Could you check a few things on this model? Use its own coordinates, in mm. A direction names the side the tool comes from. Give positions to 0.01 mm unless a question says otherwise; leave off trailing zeros. Write each loop counter-clockwise with the first axis right and the second up, starting at its lowest first coordinate (ties: lowest second). Pieces come first, ordered by that corner, then holes. Notation, with made-up numbers: M 68.25,-28 L 110.25,-28 A16 ccw 110.25,-9 Z; hole C 88.25,20 d8. An arc over 180 degrees is marked long. One line per item, written item: value.
```python
from build123d import *

# Parameters (mm, degrees)
BOSS_EXTRUDE1_DEPTH      = 180
SKETCH3_W                = 116.5
SKETCH3_H                = 142
CUT_REVOLVE1_ANGLE       = 271
WRAP1_SECTION_W          = 10
WRAP1_SECTION_H          = 10
WRAP1_ANGLE              = 2.220766648
WRAP1_SECTOR_2_SECTION_W = 10
WRAP1_SECTOR_2_SECTION_H = 10
WRAP1_SECTOR_2_ANGLE     = 2.220766648
MIRROR1_START            = 60
MIRROR1_DEPTH            = 10
MIRROR1_START_2          = 110
MIRROR1_2_DEPTH          = 10
CUT_EXTRUDE6_DEPTH       = 262.461278204
CUT_EXTRUDE6_DEPTH_BACK  = 20
SKETCH17_R               = 2
CUT_EXTRUDE7_DEPTH       = 10
CUT_EXTRUDE9_DEPTH       = 262.461278204
CUT_EXTRUDE9_DEPTH_BACK  = 262.461278204
SKETCH19_W               = 258
SKETCH19_H               = 15.225908702
CUT_EXTRUDE10_DEPTH      = 252.222015682
CUT_EXTRUDE10_DEPTH_BACK = 252.222015682
SKETCH22_W               = 258
SKETCH22_H               = 14
SKETCH22_H_2             = 3.774091298


# Read off the part's stored shape, not the designer's step: Mirror1
with BuildPart() as part:
    # Sketch1 → Boss-Extrude1 (new body)
    with BuildSketch(Plane(origin=(0, 0, 0), x_dir=(1, 0, 0), z_dir=(0, 1, 0))):
        with BuildLine():
            Line((0, -129), (0, 129))
            ThreePointArc((0, 129), (-129, 0), (0, -129))
        make_face()
    extrude(amount=BOSS_EXTRUDE1_DEPTH)

    # Sketch3 → Cut-Revolve1 (revolve, cut)
    with BuildSketch(Plane(origin=(0, 0, 0), x_dir=(0, 0, -1), z_dir=(1, 0, 0))):
        with Locations((-58.25, 90)):
            Rectangle(SKETCH3_W, SKETCH3_H)
    revolve(axis=Axis((0, 180, 0), (0, -1, 0)), revolution_arc=CUT_REVOLVE1_ANGLE, mode=Mode.SUBTRACT)

    # Wrap1 section (on wrap section) → Wrap1 (revolve)
    with BuildSketch(Plane(origin=(0, 0, 0), x_dir=(0, 0, 1), z_dir=(1, 0, 0))):
        with Locations((134, -115)):
            Rectangle(WRAP1_SECTION_W, WRAP1_SECTION_H)
    revolve(axis=Axis((0, 0, 0), (0, -1, 0)), revolution_arc=WRAP1_ANGLE)

    # Wrap1 sector 2 section (on wrap section) → Wrap1 sector 2 (revolve)
    with BuildSketch(Plane(origin=(0, 0, 0), x_dir=(0, 0, 1), z_dir=(1, 0, 0))):
        with Locations((134, -65)):
            Rectangle(WRAP1_SECTOR_2_SECTION_W, WRAP1_SECTOR_2_SECTION_H)
    revolve(axis=Axis((0, 0, 0), (0, -1, 0)), revolution_arc=WRAP1_SECTOR_2_ANGLE)

    # Mirror1 outline → Mirror1 (add)
    with BuildSketch(Plane(origin=(0, 0, 0), x_dir=(1, 0, 0), z_dir=(0, 1, 0)).offset(MIRROR1_START)):
        with BuildLine():
            ThreePointArc((0, 139), (-2.693629831, 138.973898119), (-5.386248024, 138.895602278))
            Line((-5.386248024, 138.895602278), (-4.998748166, 128.903112906))
            ThreePointArc((-4.998748166, 128.903112906), (-2.499843512, 128.975775952), (0, 129))
            Line((0, 129), (0, 139))
        make_face()
    extrude(amount=MIRROR1_DEPTH)

    # Mirror1 2 outline → Mirror1 2 (add)
    with BuildSketch(Plane(origin=(0, 0, 0), x_dir=(1, 0, 0), z_dir=(0, 1, 0)).offset(MIRROR1_START_2)):
        with BuildLine():
            ThreePointArc((0, 139), (-2.693629831, 138.973898119), (-5.386248024, 138.895602278))
            Line((-5.386248024, 138.895602278), (-4.998748166, 128.903112906))
            ThreePointArc((-4.998748166, 128.903112906), (-2.499843512, 128.975775952), (0, 129))
            Line((0, 129), (0, 139))
        make_face()
    extrude(amount=MIRROR1_2_DEPTH)

    # Sketch16 → Cut-Extrude6 (cut, two sides: drawn at the far end of the back side and taken through both)
    with BuildSketch(Plane(origin=(0, 180, 0), x_dir=(1, 0, 0), z_dir=(0, 1, 0)).offset(-CUT_EXTRUDE6_DEPTH_BACK)):
        with BuildLine():
            Line((0, 100), (0, -100))
            ThreePointArc((0, -100), (-100, 0), (0, 100))
        make_face()
    extrude(amount=CUT_EXTRUDE6_DEPTH + CUT_EXTRUDE6_DEPTH_BACK, mode=Mode.SUBTRACT)

    # Sketch17 → Cut-Extrude7 (cut)
    with BuildSketch(Plane(origin=(0, 0, 0), x_dir=(0, 0, -1), z_dir=(1, 0, 0))):
        with Locations((-134, 115)):
            Circle(SKETCH17_R)
        with Locations((-134, 65)):
            Circle(SKETCH17_R)
        with Locations(Location((134, 115, 0), (0, 0, 180))):
            Circle(SKETCH17_R)
        with Locations((134, 65)):
            Circle(SKETCH17_R)
    extrude(amount=-CUT_EXTRUDE7_DEPTH, mode=Mode.SUBTRACT)

    # Sketch19 → Cut-Extrude9 (cut, two sides: drawn at the far end of the back side and taken through both)
    with BuildSketch(Plane(origin=(0, 0, 0), x_dir=(0, 0, -1), z_dir=(1, 0, 0)).offset(-CUT_EXTRUDE9_DEPTH_BACK)):
        with Locations((0, 172.387045649)):
            Rectangle(SKETCH19_W, SKETCH19_H)
    extrude(amount=CUT_EXTRUDE9_DEPTH + CUT_EXTRUDE9_DEPTH_BACK, mode=Mode.SUBTRACT)

    # Sketch22 → Cut-Extrude10 (cut, two sides: drawn at the far end of the back side and taken through both)
    with BuildSketch(Plane(origin=(0, 0, 0), x_dir=(0, 0, -1), z_dir=(1, 0, 0)).offset(-CUT_EXTRUDE10_DEPTH_BACK)):
        with Locations((0, 7)):
            Rectangle(SKETCH22_W, SKETCH22_H)
        with Locations((0, 162.887045649)):
            Rectangle(SKETCH22_W, SKETCH22_H_2)
    extrude(amount=CUT_EXTRUDE10_DEPTH + CUT_EXTRUDE10_DEPTH_BACK, mode=Mode.SUBTRACT)


solid = part.part
```
1) Please list where these lines run through material, in increasing order: L1, parallel to Y at x = -3, z = 134; L2, parallel to Z at x = -3.1, y = 65; L3, parallel to Y at x = -89, z = 31.5. Write a range as from..to.
Outcome:
L1: y = 60..63, 67..70, 110..113, 117..120
L2: z = -138.97..-136, -132..-116.46, 116.46..132, 136..138.97
L3: y = 14..19
2) We'd pull the mould along Y, two halves only. Please class faces 4 (the face through (-3, 70, -134)), 5 (the face through (-116.47, 90.99, 2.56)), 6 (the face through (-3, 60, 134)): pulls with the +Y half, pulls with the -Y half, needs draft (parallel to the pull), parting line crosses it, or undercut.
Outcome:
face 4: undercut
face 5: needs draft
face 6: pulls with the -Y half
3) If we section it at B-B, the plane z = 0: Write out the boundary of the cut face in (x, y).
Outcome:
outline: M -129,14 L 0,14 L 0,19 L -116.5,19 L -116.5,161 L -129,161 Z
4) On a 3-axis mill with a long thin cutter (end or side, diameter ignored), from which of +Z, -Z, +X, -X, +Y, -Y can I reach the whole of each face in a straight line? I mean faces 1 (the face through (-5.104, 114.93, 131.609)), 2 (the face through (-3, 60, -134)), 3 (the face through (-3, 70, 134)). Say none if no direction works.
Outcome:
face 1: -X, +Y, -Y
face 2: -Z, +X, -X, -Y
face 3: +Z, +X, -X
5) I'm going to push flat-ended pins straight in: pin 1 (1.6 mm diameter, centred on x = -3, z = 135, fed in from +Y); pin 2 (3.5 mm diameter, centred on y = 115, z = 134, fed in from +X); pin 3 (4 mm diameter, centred on y = 89, z = -24.5, fed in from -X); pin 4 (6 mm diameter, centred on x = -3, z = -133.5, fed in from -Y). Where does each tip first touch, or does it pass through?
Outcome:
pin 1: stops at y = 120
pin 2: passes through
pin 3: stops at x = -127.02
pin 4: stops at y = 60
6) If we section it at D-D, the plane x = -59: Write out the boundary of the cut face in (y, z), then the cut area to 3 significant figures.
Outcome:
outline: M 14,-114.72 L 161,-114.72 L 161,-100.46 L 19,-100.46 L 19,100.46 L 161,100.46 L 161,114.72 L 14,114.72 Z
area: 5,200 mm^2
7) If we section it at A-A, the plane x = -74.5: Write out the boundary of the cut face in (y, z), then the cut area to 3 significant figures.
Outcome:
outline: M 14,-105.31 L 161,-105.31 L 161,-89.57 L 19,-89.57 L 19,89.57 L 161,89.57 L 161,105.31 L 14,105.31 Z
area: 5,530 mm^2
8) If we section it at C-C, the plane y = 125: Write out the boundary of the cut face in (x, z).
Outcome:
outline: M 0,-129 L 0,-116.5 A116.5 cw 0,116.5 L 0,129 A129 ccw Z
